```python
from build123d import *

# Parameters (mm, degrees)
BOSS_EXTRUDE1_DEPTH = 1.524


with BuildPart() as part:
    # Sketch1 → Boss-Extrude1 (new body)
    with BuildSketch(Plane(origin=(0, 0, 0), x_dir=(1, 0, 0), z_dir=(0, 1, 0))):
        with BuildLine():
            Line((0, 1.651), (1.778, 1.651))
            Line((1.778, 1.651), (1.778, 3.369690787))
            ThreePointArc((1.778, 3.369690787), (-3.81, 0), (1.778, -3.369690787))
            Line((1.778, -3.369690787), (1.778, -1.651))
            Line((1.778, -1.651), (0, -1.651))
            ThreePointArc((0, -1.651), (-1.651, 0), (0, 1.651))
        make_face()
    extrude(amount=BOSS_EXTRUDE1_DEPTH)


solid = part.part
```
Can you work these out from the model? Positions are in its coordinate system, mm. A direction names the side the tool comes from. Coordinates: 2 decimals unless noted, no trailing zeros. Write each loop counter-clockwise with the first axis right and the second up, starting at its lowest first coordinate (ties: lowest second). Pieces come first, ordered by that corner, then holes. Notation, with made-up numbers: (75.5, 1.5) - (83.5, 1.5) arc R32 cw to (83.5, 32.5) - close; hole circle Ø9 at (17.25, -36). An arc over 180 degrees is marked (long way). Return JSON: item names as keys, results as strings.
Q1. If we section it at A-A (x = -1.3): Please give me the cut outline in (y, z), then the cut area to 3 significant figures.
Computed values:
{"outline": "(0, -3.58) - (1.52, -3.58) - (1.52, -1.02) - (0, -1.02) - close; (0, 1.02) - (1.52, 1.02) - (1.52, 3.58) - (0, 3.58) - close", "area": "7.81 mm2"}
Q2. Thinking about a two-plate mould opening in Z: for faces 1 (the flat face through (1, 1, -1.651)), 2 (the flat face through (1.778, 1, -2)), 3 (the cylindrical face through (-3.81, 0.75, -0.11)), which applies, +Z half, -Z half, draft (parallel to the pull), parting line (faces both ways), or undercut?
Computed values:
{"face 1": "undercut", "face 2": "draft", "face 3": "parting line"}
Q3. If we section it at D-D (x = 0.55): Please give me the cut outline in (y, z).
Computed values:
{"outline": "(0, -3.77) - (1.52, -3.77) - (1.52, -1.65) - (0, -1.65) - close; (0, 1.65) - (1.52, 1.65) - (1.52, 3.77) - (0, 3.77) - close"}
Q4. I'm going to push a flat-ended pin straight in: pin 1 Ø0.5 at (x, y) = (0.5, 1) entering from +Z. Where does the tip first touch, or does it pass through?
Computed values:
{"pin 1": "stops at z = 3.8"}
Q5. On a 3-axis mill with a long thin cutter (end or side, diameter ignored), from which of +Z, -Z, +X, -X, +Y, -Y can I reach the whole of each face in a straight line? I mean faces 4 (the flat face through (1, 1, 1.651)), 5 (the flat face through (1.778, 1, 3)). Say none if no direction works.
Computed values:
{"face 4": "+X, +Y, -Y", "face 5": "+Z, -Z, +X, +Y, -Y"}
Q6. Please list where these lines run through material, in increasing order: L1, parallel to Z at x = 0.4, y = 1.2; L2, parallel to Z at x = -0.4, y = 1.05; L3, parallel to X at y = 0.95, z = 0.75. Write a range as from..to.
Computed values:
{"L1": "z = -3.79..-1.65, 1.65..3.79", "L2": "z = -3.79..-1.6, 1.6..3.79", "L3": "x = -3.74..-1.47"}
Q7. If we section it at C-C (z = 0): Please give me the cut outline in (x, y).
Computed values:
{"outline": "(-3.81, 0) - (-1.65, 0) - (-1.65, 1.52) - (-3.81, 1.52) - close"}
Q8. If we section it at B-B (y = 1.05): Please give me the cut outline in (x, z).
Computed values:
{"outline": "(0, -1.65) arc R1.65 cw to (0, 1.65) - (1.78, 1.65) - (1.78, 3.37) arc R3.81 ccw (long way) to (1.78, -3.37) - (1.78, -1.65) - close"}
